Source: CAD feature listing. Evaluate the final solid. Frame: model axes, mm. A direction names the side the tool comes from. Round coordinates to 2 decimals unless told otherwise and drop trailing zeros. Write each loop counter-clockwise with the first axis right and the second up, starting at its lowest first coordinate (ties: lowest second). Pieces come first, ordered by that corner, then holes. Notation, with made-up numbers: M 74,45 L 96,45 A21 ccw 96,73 Z; hole C -35,28.25 d5. An arc over 180 degrees is marked long. Use a Markdown table: item, result.
```python
from build123d import *

# Parameters (mm, degrees)
BOSS_EXTRUDE1_DEPTH     = 2.5
SKETCH4_W               = 41.785
SKETCH4_H               = 150
CUT_EXTRUDE1_DEPTH      = 120
SKETCH5_W               = 5
SKETCH5_H               = 60
BOSS_EXTRUDE2_DEPTH     = 22.5
CUT_EXTRUDE2_DEPTH      = 106.948100502
CUT_EXTRUDE2_DEPTH_BACK = 106.948100502
SKETCH3_R               = 15
SKETCH3_R_2             = 18


with BuildPart() as part:
    # Sketch2 → Boss-Extrude1 (new, symmetric)
    with BuildSketch(Plane(origin=(0, 0, 0), x_dir=(1, 0, 0), z_dir=(0, 1, 0))):
        with BuildLine():
            Line((-26.65, 80), (-76.785, 80))
            Line((-76.785, 80), (-76.785, -70))
            Line((-76.785, -70), (76.785, -70))
            Line((76.785, -70), (76.785, 80))
            Line((76.785, 80), (26.65, 80))
            Line((26.65, 80), (26.65, 75.5))
            Line((26.65, 75.5), (27.4, 75.5))
            ThreePointArc((27.4, 75.5), (25, 73.1), (22.6, 75.5))
            Line((22.6, 75.5), (23.35, 75.5))
            Line((23.35, 75.5), (23.35, 80))
            Line((23.35, 80), (-23.35, 80))
            Line((-23.35, 80), (-23.35, 75.5))
            Line((-23.35, 75.5), (-22.6, 75.5))
            ThreePointArc((-22.6, 75.5), (-25, 73.1), (-27.4, 75.5))
            Line((-27.4, 75.5), (-26.65, 75.5))
            Line((-26.65, 75.5), (-26.65, 80))
        make_face()
    extrude(amount=BOSS_EXTRUDE1_DEPTH, both=True)

    # Sketch4 → Cut-Extrude1 (cut)
    with BuildSketch(Plane(origin=(0, 2.5, 0), x_dir=(1, 0, 0), z_dir=(0, 1, 0))):
        with Locations((-55.8925, 5)):
            Rectangle(SKETCH4_W, SKETCH4_H)
        with Locations((55.8925, 5)):
            Rectangle(SKETCH4_W, SKETCH4_H)
    extrude(amount=-CUT_EXTRUDE1_DEPTH, mode=Mode.SUBTRACT)

    # Sketch5 → Boss-Extrude2 (add, symmetric)
    with BuildSketch(Plane(origin=(0, 0, 0), x_dir=(0, 0, -1), z_dir=(1, 0, 0))):
        with Locations((-72.5, -27.5)):
            Rectangle(SKETCH5_W, SKETCH5_H)
    extrude(amount=BOSS_EXTRUDE2_DEPTH, both=True)

    # Sketch3 → Cut-Extrude2 (cut, two sides: drawn at the far end of the back side and taken through both)
    with BuildSketch(Plane(origin=(0, 2.5, 0), x_dir=(1, 0, 0), z_dir=(0, 1, 0)).offset(-CUT_EXTRUDE2_DEPTH_BACK)):
        with Locations(Location((0, 44, 0), (0, 0, 270))):
            Circle(SKETCH3_R)
        with Locations(Location((0, -51, 0), (0, 0, 270))):
            Circle(SKETCH3_R)
        with Locations(Location((0, 0, 0), (0, 0, 270))):
            Circle(SKETCH3_R_2)
    extrude(amount=CUT_EXTRUDE2_DEPTH + CUT_EXTRUDE2_DEPTH_BACK, mode=Mode.SUBTRACT)


solid = part.part
```
Q1. Section D-D on y = -44.5. Return loops of the section in (x, z).
Results are:
| item | result |
|---|---|
| outline | M -22.5,70 L 22.5,70 L 22.5,75 L -22.5,75 Z |
Q2. Section C-C on z = -44. Return loops of the section in (x, y), plus the area to 3 significant figures.
Results are:
| item | result |
|---|---|
| outline | M -35,-2.5 L -15,-2.5 L -15,2.5 L -35,2.5 Z; M 15,-2.5 L 35,-2.5 L 35,2.5 L 15,2.5 Z |
| area | 200 mm^2 |
Q3. Reachability of faces 1 (the flat face through (0, -2.5, -23)), 2 (the flat face through (29, 0, 70)), 3 (the flat face through (0, -28, 75)), 4 (the flat face through (-23.35, 0, -78)) from +Z, -Z, +X, -X, +Y, -Y: full face, straight path, thin tool, end or side. Return the list, or none.
Results are:
| item | result |
|---|---|
| face 1 | -Z, +X, -X, -Y |
| face 2 | +Z, +X, +Y, -Y |
| face 3 | +Z, +X, -X, +Y, -Y |
| face 4 | -Z, +Y, -Y |
Q4. Section A-A on z = 0. Return loops of the section in (x, y), plus the area to 3 significant figures.
Results are:
| item | result |
|---|---|
| outline | M -35,-2.5 L -18,-2.5 L -18,2.5 L -35,2.5 Z; M 18,-2.5 L 35,-2.5 L 35,2.5 L 18,2.5 Z |
| area | 170 mm^2 |
Q5. Mould query, pull axis X, two halves, no side actions, for faces 5 (the flat face through (35, 0, -4)), 6 (the flat face through (-35, 0, -4)), 7 (the cylindrical face through (0.66, -0.035, 36.015)), 8 (the flat face through (-29, 0, 70)). Classes: +X half, -X half, draft (parallel to the pull), parting line (faces both ways), or undercut.
Results are:
| item | result |
|---|---|
| face 5 | +X half |
| face 6 | -X half |
| face 7 | undercut |
| face 8 | draft |
Q6. Line query: L1, parallel to Z at x = 0, y = 1; L2, parallel to X at y = 0.3, z = 0; L3, parallel to X at y = 0.95, z = 51. Output: solid intervals per line, ascending.
Results are:
| item | result |
|---|---|
| L1 | -80 to -59, -29 to -18, 18 to 36, 66 to 75 |
| L2 | -35 to -18, 18 to 35 |
| L3 | -35 to -15, 15 to 35 |
Q7. Section B-B on x = 0. Return loops of the section in (y, z), plus the area to 3 significant figures.
Results are:
| item | result |
|---|---|
| outline | M -57.5,70 L -2.5,70 L -2.5,66 L 2.5,66 L 2.5,75 L -57.5,75 Z; M -2.5,-80 L 2.5,-80 L 2.5,-59 L -2.5,-59 Z; M -2.5,-29 L 2.5,-29 L 2.5,-18 L -2.5,-18 Z; M -2.5,18 L 2.5,18 L 2.5,36 L -2.5,36 Z |
| area | 570 mm^2 |
Q8. First-contact query: pin 1 Ø2.5 at (x, y) = (-30.5, 0.5) entering from +Z; pin 2 Ø6 at (x, y) = (6, -31) entering from -Z; pin 3 Ø1.5 at (y, z) = (-38, 71.5) entering from +X. Flat tips, straight axial feed; report the tip coordinate or a pass-through.
Results are:
| item | result |
|---|---|
| pin 1 | z = 70 |
| pin 2 | z = 70 |
| pin 3 | x = 22.5 |
